Geometry: final body of the model. Coordinates: model frame, mm. A direction names the side the tool comes from. Give positions to 0.01 mm unless a question says otherwise; leave off trailing zeros. Write each loop counter-clockwise with the first axis right and the second up, starting at its lowest first coordinate (ties: lowest second). Pieces come first, ordered by that corner, then holes.
Q1. Reachability of faces 4 (the flat face through (0, 0, 0)), 5 (the cylindrical face through (-2.38, 3.26, 13.03)) from +Z, -Z, +X, -X, +Y, -Y: full face, straight path, thin tool, end or side. Return the list, or none.
Q2. Section C-C (x = 12). Return the cut outline in (y, z).
Q3. Section B-B (z = -9). Return the cut outline in (x, y).
Q4. Line query: line 1 (Z direction, x = -12, y = 9.75); line 2 (X direction, y = 8, z = 9); line 3 (X direction, y = 15, z = -9). Output: solid intervals per line, ascending.
Q5. Mould query, pull axis X, two halves, no side actions, for faces 1 (the cylindrical face through (-1.08, 9.12, -1.82)), 2 (the flat face through (17.5, 14, 0)), 3 (the flat face through (-17.5, 14, 0)). Classes: +X half, -X half, draft (parallel to the pull), parting line (faces both ways), or undercut.
Q6. Section A-A (y = 14). Return the cut outline in (x, z).
Q7. Section D-D (y = 24.25). Return the cut outline in (x, z), plus the area to 3 significant figures.
Q8. Pin query (flat end, axial travel): pin 1 Ø11 at (x, y) = (4, 14) entering from +Z. Return the tip coordinate at first contact, or that it passes through.
from build123d import *

# Parameters (mm, degrees)
SKETCH1_W           = 35
SKETCH1_H           = 30
SKETCH1_R           = 2
BOSS_EXTRUDE1_DEPTH = 28
SKETCH2_R           = 11
CUT_EXTRUDE1_DEPTH  = 4
SKETCH3_R           = 5
CUT_EXTRUDE2_DEPTH  = 27


with BuildPart() as part:
    # Sketch1 → Boss-Extrude1 (new body)
    with BuildSketch(Plane(origin=(0, 0, 0), x_dir=(1, 0, 0), z_dir=(0, 1, 0))):
        Rectangle(SKETCH1_W, SKETCH1_H)
        with Locations((-12, 9)):
            Circle(SKETCH1_R, mode=Mode.SUBTRACT)
        with Locations((-12, -9)):
            Circle(SKETCH1_R, mode=Mode.SUBTRACT)
        with Locations((12, -9)):
            Circle(SKETCH1_R, mode=Mode.SUBTRACT)
        with Locations((12, 9)):
            Circle(SKETCH1_R, mode=Mode.SUBTRACT)
    extrude(amount=BOSS_EXTRUDE1_DEPTH)

    # Sketch2 → Cut-Extrude1 (cut)
    with BuildSketch(Plane.XY.offset(15)):
        with Locations((0, 14)):
            Circle(SKETCH2_R)
    extrude(amount=-CUT_EXTRUDE1_DEPTH, mode=Mode.SUBTRACT)

    # Sketch3 → Cut-Extrude2 (cut, through all)
    with BuildSketch(Plane.XY.offset(11)):
        with Locations((0, 14)):
            Circle(SKETCH3_R)
    extrude(amount=-CUT_EXTRUDE2_DEPTH, mode=Mode.SUBTRACT)


solid = part.part
Computed:
1. face 4: +Z, -Z, +X, -X, -Y
1. face 5: +Z
2. outline: (0, -15) - (28, -15) - (28, -11) - (0, -11) - close; (0, -7) - (28, -7) - (28, 7) - (0, 7) - close; (0, 11) - (28, 11) - (28, 15) - (0, 15) - close
3. outline: (-17.5, 0) - (-14, 0) - (-14, 28) - (-17.5, 28) - close; (-10, 0) - (10, 0) - (10, 28) - (-10, 28) - close; (14, 0) - (17.5, 0) - (17.5, 28) - (14, 28) - close; hole circle Ø10 at (0, 14)
4. line 1: z = -15 to -11, -7 to 7, 11 to 15
4. line 2: x = -17.5 to -14, -10 to 10, 14 to 17.5
4. line 3: x = -17.5 to -14, -10 to -4.9, 4.9 to 10, 14 to 17.5
5. face 1: undercut
5. face 2: +X half
5. face 3: -X half
6. outline: (-17.5, -15) - (-5, -15) - (-5, 11) - (-11, 11) - (-11, 15) - (-17.5, 15) - close; (5, -15) - (17.5, -15) - (17.5, 15) - (11, 15) - (11, 11) - (5, 11) - close; hole circle Ø4 at (-12, -9); hole circle Ø4 at (-12, 9); hole circle Ø4 at (12, -9); hole circle Ø4 at (12, 9)
7. outline: (-17.5, -15) - (17.5, -15) - (17.5, 15) - (3.99, 15) - (3.99, 11) - (-3.99, 11) - (-3.99, 15) - (-17.5, 15) - close; hole circle Ø4 at (-12, -9); hole circle Ø4 at (-12, 9); hole circle Ø4 at (12, -9); hole circle Ø4 at (12, 9)
7. area: 968 mm2
8. pin 1: stops at z = 11
